Part model, mm, in its own coordinate system. Face numbers are marked on the shaded views. A direction names the side the tool comes from. Give positions to 0.01 mm unless a question says otherwise; leave off trailing zeros. Use CSV: the item, a comma, the result in double quotes. Start each with the question number.
Item 1: Drill centre lines: line 1 (Z direction, x = 1.85, y = 5); line 2 (Z direction, x = 20.5, y = 1.25); line 3 (X direction, y = 1.75, z = 12). Where is each one in solid material? Low to high. Write a range as [from, to].
Item 2: Mould opens along X. For the marked faces 1, 2 and 3 say: released by +X, released by -X, zero draft, split by the parting line, or undercut.
Item 3: Pin check, flat tips, straight feed: pin 1 (2 mm diameter, centred on y = 5, z = 14, fed in from -X); pin 2 (2 mm diameter, centred on x = 2, y = 5, fed in from +Z); pin 3 (1 mm diameter, centred on x = 14.5, y = 4.5, fed in from -Z). Stop position of each tip, or through.
Item 4: Cut at A-A (z = 14). Count the separate pieces of the cut face and the enclosed holes in it, then the cut area to 3 significant figures.
Item 5: Which spindle directions (+Z, -Z, +X, -X, +Y, -Y) get a long thin tool onto all of the face, cutting with end or side? Do the marked faces 4 and 5. Say none if no direction does.
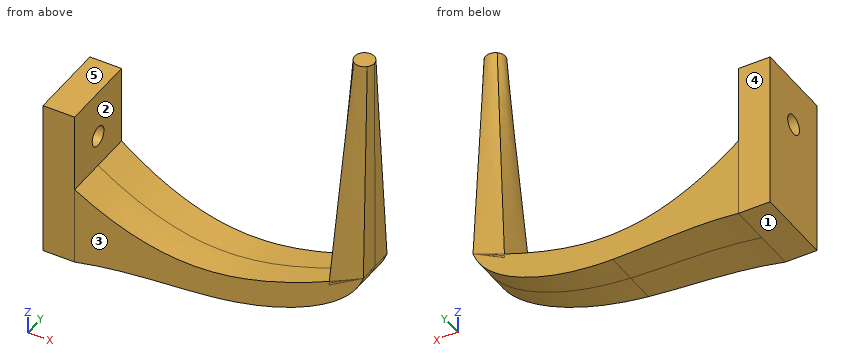
Autodesk Fusion 360 part; units mm, degrees
sketch "Sketch1" plane through (0, 0, 0) normal (1, 0, 0) x (0, 1, 0)
  line L0 (0, 0) -> (10, 0)
  line L1 (10, 0) -> (10, 20)
  line L2 (10, 20) -> (0, 20)
  line L3 (0, 20) -> (0, 0)
  circle A0 centre (5, 14) radius 1.25
  line L4 (5, 20) -> (5, 0) construction
  dimension "d1" = 10
  dimension "d2" = 20
  dimension "d3" = 6
  dimension "d4" = 2.5
extrude "Extrude1" add sketch "Sketch1" along normal blind 4
ref_plane "WorkPlane1" through (0, 5, 0) normal (0, 1, 0) x (0, 0, 1)
sketch "Sketch2" plane through (0, 5, 0) normal (0, 1, 0) x (1, 0, 0)
  spline S0 degree 5 poles (4, 0) (4.5771, -0.1055) (5.7551, -0.2992) (7.5934, -0.5374) (10.1902, -0.7501) (13.6911, -0.8547) (17.4735, -0.8864) (21.5365, -0.9956) (25.924, -1.5675) (30.3819, -2.7889) (34.4435, -4.6461) (36.9623, -6.5714) (38.2422, -8.2146) (38.7971, -9.3913) (39, -10) knots 0 0 0 0 0 0 0.1 0.2 0.3 0.4 0.5 0.6 0.7 0.8 0.9 1 1 1 1 1 1
  line L0 (15.7367, -0.7193) -> (25.4307, -1.3448)
  line L1 (0, 0) -> (4, 0)
  line L2 (38, -7) -> (40, -13)
  spline S1 degree 5 poles (39, -10) (38.7242, -9.8626) (38.1556, -9.5847) (37.2514, -9.1586) (35.9422, -8.5717) (34.1308, -7.8106) (32.1444, -7.0347) (29.9895, -6.2707) (27.6837, -5.5654) (25.2519, -4.9777) (22.7222, -4.5714) (20.1223, -4.4064) (17.4768, -4.5309) (14.8034, -4.9704) (12.1137, -5.7332) (9.4148, -6.8176) (7.2511, -7.9369) (5.6263, -8.915) (4.5423, -9.6281) (4, -10) knots 0 0 0 0 0 0 0.066667 0.133333 0.2 0.266667 0.333333 0.4 0.466667 0.533333 0.6 0.666667 0.733333 0.8 0.866667 0.933333 1 1 1 1 1 1
  line L3 (4, 0) -> (4, -10)
  line L4 (39, -10) -> (30.4055, -5.1224)
  point P0 (20.5837, -1.0321)
  point P1 (32, -7)
  point P2 (19.692, -4.4795)
  dimension "d8" = 35
  dimension "d9" = 10
  dimension "d10" = 4
  dimension "d11" = 10
extrude "Extrude2" add sketch "Sketch2" along normal mid plane 10
sketch "Sketch3" plane through (0, 0, 0) normal (0, 0, -1) x (1, 0, 0)
  line L0 (0, 0) -> (0, -10)
  line L1 (0, -10) -> (4, -10)
  line L2 (4, -10) -> (4, 0)
  line L3 (4, 0) -> (0, 0)
  line L4 (4, -10) -> (39.3, -7.5414)
  line L5 (39.3, -7.5414) -> (39.3, -2.5414)
  line L6 (39.3, -2.5414) -> (4, 0)
  line L7 (4, -10) -> (44.4178, -17.1605)
  line L8 (44.4178, -17.1605) -> (44.4178, 8.7922)
  line L9 (44.4178, 8.7922) -> (4, 0)
  dimension "d16" = 5
  dimension "d17" = 35.3
extrude "Extrude3" cut sketch "Sketch3" against normal blind 15 contours L4 L5 L6 L7 L8 L9
ref_plane "WorkPlane2" through (39, 2.5199, 10) normal (-0.4936, 0, 0.8697) x (0, -1, 0)
sketch "Sketch4" plane through (5.2084, 0, -9.1775) normal (-0.4936, 0, 0.8697) x (0, -1, 0)
  line L0 (-7.5622, 38.8542) -> (-2.52, 38.8542)
  line L1 (-2.52, 38.8542) -> (-2.2042, 34.0638)
  line L2 (-2.2042, 34.0638) -> (-7.8675, 34.0638)
  line L3 (-7.8675, 34.0638) -> (-7.5622, 38.8542)
ref_plane "WorkPlane3" through (0, 0, 38) normal (0, 0, 1) x (1, 0, 0)
sketch "Sketch5" plane through (0, 0, 38) normal (0, 0, 1) x (1, 0, 0)
  circle A0 centre (37.674, 5.005) radius 1.25
  dimension "d25" = 2.5
loft "Loft1" add profiles "Sketch4", "Sketch5" section 1 section 2
Worked answers:
1,line 1,"z = [0, 12.75], [15.25, 20]"
1,line 2,"z = [1.03, 4.48]"
1,line 3,"x = [0, 4]"
2,face 1,"zero draft"
2,face 2,"undercut"
2,face 3,"released by +X"
3,pin 1,"stops at x = 35.11"
3,pin 2,"stops at z = 20"
3,pin 3,"stops at z = 0.84"
4,separate pieces,"3"
4,enclosed holes,"0"
4,area,"48.1 mm^2"
5,face 4,"+Z, -Z, +X, -X, +Y"
5,face 5,"+Z, -X, +Y, -Y"
